Geometry: final body of the model. Coordinates: model frame, mm. A direction names the side the tool comes from. Give positions to 0.01 mm unless a question says otherwise; leave off trailing zeros. Order: outer loops, then holes, each group sorted by start corner. A loop starts at its lowest first (then second) coordinate and runs counter-clockwise, first axis right, second up. Notation, with made-up numbers: (79, -36.75) -> (119, -36.75) arc R25 cw to (119, 0.25) -> close; hole circle Ø5 at (57, 25). An arc over 180 degrees is marked (long way). Answer in a Markdown table with one row per item. Add a question column.
Q1. Contact query for flat-ended pins moving along their axis: P1, Ø4, axis at x = 4, y = 4, coming from the -Z side; P2, Ø1, axis at x = 3.5, y = 5.5, coming from the +Z side; P3, Ø1.8, axis at x = -1, y = -8, coming from the +Z side. Output: stop coordinate, or through.
Q2. Pull-direction query (X, two-part tool) for faces 1 (the face through (-1.125, -14, 3)), 2 (the face through (0, -15.75, 2)), 3 (the face through (-3.575, -12, 3)), 4 (the face through (-7.375, 0, 1)); classes: +X half, -X half, draft (parallel to the pull), parting line (faces both ways), or undercut.
Q3. Cut plane A-A on z = 3.45. Return the cut outline in (x, y) (3 decimals), and give its area (3 significant figures).
Q4. Line query: line 1 along Y through (x, z) = (6.5, 4.15); line 2 along Y through (x, z) = (1, 3.05); line 3 along Y through (x, z) = (-4.5, 1.95). Output: solid intervals per line, ascending. Write a range as from..to.
Q5. Cut plane B-B on x = 3.5. Return the cut outline in (y, z).
Q6. Cut plane D-D on x = -4. Return the cut outline in (y, z), and give its area (3 significant figures).
Q7. Set-up query: faces 5 (the face through (3, -11.25, 3)), 6 (the face through (5, -0.15, 3)), 7 (the face through (0, -7, 1.9)). Return all of +Z, -Z, +X, -X, +Y, -Y with unobstructed straight access to the full face (end or side cutting, diameter ignored); none if empty.
Q8. Cut plane C-C on y = -1. Return the cut outline in (x, z) (3 decimals).
from build123d import *

# Parameters (mm, degrees)
F0_W     = 14.75
F0_H     = 31.5
F1_DEPTH = 1.7
F2_W     = 14.75
F2_H     = 5.35
F2_W_2   = 8.5
F2_H_2   = 4.5
F2_W_3   = 3.8
F2_H_3   = 7.6
F2_W_4   = 4.7
F2_H_4   = 7.55
F3_DEPTH = 2.9
F5_DEPTH = 0.2


with BuildPart() as f1:
    # F0 (on Top) → F1 (new body)
    with BuildSketch(Plane.XY):
        Rectangle(F0_W, F0_H)
    extrude(amount=F1_DEPTH)

    # F2 (on face) → F3 (join)
    with BuildSketch(Plane.XY.offset(1.7)):
        with Locations((0, 13.075)):
            Rectangle(F2_W, F2_H)
        with Locations((3.125, -13.5)):
            Rectangle(F2_W_2, F2_H_2)
        with Locations((-5.475, -11.95)):
            Rectangle(F2_W_3, F2_H_3)
        with Locations((5.025, -3.925)):
            Rectangle(F2_W_4, F2_H_4)
    extrude(amount=F3_DEPTH)

    # F4 (on face) → F5 (join)
    with BuildSketch(Plane.XY.offset(1.7)):
        Polygon((0.789278, -3.898788), (0, -3.898788), (-0.789278, -3.898788), (-0.789278, -6.957673), (-1.8306, -6.957673), (0, -10.08164), (1.8306, -6.957673), (0.789278, -6.957673), align=None)
    extrude(amount=F5_DEPTH)


solid = f1.part
Completed:
| question | item | result |
|---|---|---|
| 1 | P1 | stops at z = 0 |
| 1 | P2 | stops at z = 1.7 |
| 1 | P3 | stops at z = 1.9 |
| 2 | face 1 | undercut |
| 2 | face 2 | draft |
| 2 | face 3 | undercut |
| 2 | face 4 | -X half |
| 3 | outline | (-7.375, -15.75) -> (-3.575, -15.75) -> (-3.575, -8.15) -> (-7.375, -8.15) -> close; (-7.375, 10.4) -> (7.375, 10.4) -> (7.375, 15.75) -> (-7.375, 15.75) -> close; (-1.125, -15.75) -> (7.375, -15.75) -> (7.375, -11.25) -> (-1.125, -11.25) -> close; (2.675, -7.7) -> (7.375, -7.7) -> (7.375, -0.15) -> (2.675, -0.15) -> close |
| 3 | area | 182 mm² |
| 4 | line 1 | y = -15.75..-11.25, -7.7..-0.15, 10.4..15.75 |
| 4 | line 2 | y = -15.75..-11.25, 10.4..15.75 |
| 4 | line 3 | y = -15.75..-8.15, 10.4..15.75 |
| 5 | outline | (-15.75, 0) -> (15.75, 0) -> (15.75, 4.6) -> (10.4, 4.6) -> (10.4, 1.7) -> (-0.15, 1.7) -> (-0.15, 4.6) -> (-7.7, 4.6) -> (-7.7, 1.7) -> (-11.25, 1.7) -> (-11.25, 4.6) -> (-15.75, 4.6) -> close |
| 6 | outline | (-15.75, 0) -> (15.75, 0) -> (15.75, 4.6) -> (10.4, 4.6) -> (10.4, 1.7) -> (-8.15, 1.7) -> (-8.15, 4.6) -> (-15.75, 4.6) -> close |
| 6 | area | 91.1 mm² |
| 7 | face 5 | +Z, +X |
| 7 | face 6 | +Z, +X, -X |
| 7 | face 7 | +Z |
| 8 | outline | (-7.375, 0) -> (7.375, 0) -> (7.375, 4.6) -> (2.675, 4.6) -> (2.675, 1.7) -> (-7.375, 1.7) -> close |
